The listing builds one solid part. Answer for the finished solid, in the listing's coordinates (mm). A direction names the side the tool comes from. Coordinates: 2 decimals unless noted, no trailing zeros. Order: outer loops, then holes, each group sorted by start corner. A loop starts at its lowest first (then second) coordinate and runs counter-clockwise, first axis right, second up. Notation, with made-up numbers: (85, 88.25) -> (140, 88.25) arc R25 cw to (140, 118.25) -> close; hole circle Ø8 at (64.25, 33). An arc over 180 degrees is marked (long way). Return JSON: item names as keys, results as strings.
from build123d import *

# Parameters (mm, degrees)
F1_DEPTH = 60
F2_SIZE  = 18
F4_DEPTH = 50
F6_W     = 58.8767696172
F6_H     = 9.2865563929
F7_DEPTH = 90
F8_W     = 55
F8_H     = 5
F9_DEPTH = 100


with BuildPart() as f1:
    # F0 (on Top) → F1 (new body)
    with BuildSketch(Plane.XY):
        Polygon((-16.9115909807, -35.1172805215), (16.9115909807, -35.1172805215), (38, -8.6732520268), (30.4736339606, 24.3019121461), (0, 38.9772408044), (-30.4736339606, 24.3019121461), (-38, -8.6732520268), align=None)
    extrude(amount=F1_DEPTH)

    # F2
    f2_edges = [f1.edges().sort_by_distance(p)[0] for p in [
        (0, -35.117281, 0),
        (27.455795, -21.895266, 0),
        (34.236817, 7.81433, 0),
        (15.236817, 31.639576, 0),
        (-15.236817, 31.639576, 0),
        (-34.236817, 7.81433, 0),
        (-27.455795, -21.895266, 0),
        (0, -35.117281, 60),
        (27.455795, -21.895266, 60),
        (34.236817, 7.81433, 60),
        (15.236817, 31.639576, 60),
        (-15.236817, 31.639576, 60),
        (-34.236817, 7.81433, 60),
        (-27.455795, -21.895266, 60),
    ]]
    chamfer(f2_edges, length=F2_SIZE)

    # F3 (on face) → F4 (cut)
    with BuildSketch(Plane.XY.offset(60)):
        Polygon((-18.5224097697, -4.2276191599), (-8.2432478421, -17.1172805215), (8.2432478421, -17.1172805215), (18.5224097697, -4.2276191599), (14.8538193524, 11.8455256568), (0, 18.9987480492), (-14.8538193524, 11.8455256568), align=None)
    extrude(amount=-F4_DEPTH, mode=Mode.SUBTRACT)

    # F6 (on offset) → F7 (cut)
    with BuildSketch(Plane.XZ.offset(45)):
        with Locations((0.9286543354, 60.4554843158)):
            Rectangle(F6_W, F6_H)
    extrude(amount=-F7_DEPTH, mode=Mode.SUBTRACT)

    # F8 (on offset) → F9 (cut)
    with BuildSketch(Plane.XZ.offset(45)):
        with Locations((3.5671484997, 2.5)):
            Rectangle(F8_W, F8_H)
    extrude(amount=-F9_DEPTH, mode=Mode.SUBTRACT)


solid = f1.part
1. The part is cut by section C-C on y = 7.5. Give the vertices of the cut face in (x, z).
Answer block:
{"outline": "(-34.31, 18) -> (-20.97, 5) -> (20.97, 5) -> (34.31, 18) -> (34.31, 42) -> (20.14, 55.81) -> (15.85, 55.81) -> (15.85, 10) -> (-15.85, 10) -> (-15.85, 55.81) -> (-20.14, 55.81) -> (-34.31, 42) -> close"}
2. For faces 1 (the face through (0, -17.117, 33)), 2 (the face through (22.16, -17.97, 11.41)), determine the directions among +Z, -Z, +X, -X, +Y, -Y from which every point of the face is accessible in a straight line to the end or side of a thin tool.
Answer block:
{"face 1": "+Z", "face 2": "-Z, +X, -Y"}
3. Consider line 1 (Z direction, x = -8, y = 1.5); line 2 (X direction, y = 6, z = 12); line 3 (X direction, y = 5.5, z = 16.5). Determine where each line is inside the solid, lowest interval first. Write a range as from..to.
Answer block:
{"line 1": "z = 5..10", "line 2": "x = -28.5..-16.19, 16.19..28.5", "line 3": "x = -33.23..-16.3, 16.3..33.23"}
4. The part is cut by section A-A on z = 30. Give the vertices of the cut face in (x, y), and give its area (3 significant figures).
Answer block:
{"outline": "(-38, -8.67) -> (-16.91, -35.12) -> (16.91, -35.12) -> (38, -8.67) -> (30.47, 24.3) -> (0, 38.98) -> (-30.47, 24.3) -> close; hole (-18.52, -4.23) -> (-8.24, -17.12) -> (8.24, -17.12) -> (18.52, -4.23) -> (14.85, 11.85) -> (0, 19) -> (-14.85, 11.85) -> close", "area": "3,170 mm2"}
5. Determine the mould class of faces 3 (the face through (15.45, 31.537, 29.832)), 4 (the face through (7.531, 15.372, 33.227)), 5 (the face through (0, 1, 5)) for opening direction X: pulls with the +X half, pulls with the -X half, needs draft (parallel to the pull), parting line crosses it, or undercut.
Answer block:
{"face 3": "pulls with the +X half", "face 4": "undercut", "face 5": "needs draft"}
6. The part is cut by section D-D on z = 9. Give the vertices of the cut face in (x, y).
Answer block:
{"outline": "(-28.26, -6.45) -> (-12.58, -26.12) -> (12.58, -26.12) -> (28.26, -6.45) -> (22.66, 18.07) -> (0, 28.99) -> (-22.66, 18.07) -> close"}
7. Each of these flat-tipped pins is pushed along its axis until it touches: pin 1 Ø18 at (x, y) = (-2, -4.5) entering from +Z; pin 2 Ø5 at (y, z) = (-27, 12) entering from +X; pin 3 Ø8 at (x, y) = (27.5, -22) entering from +Z. Where does it stop, or does it pass through?
Answer block:
{"pin 1": "stops at z = 10", "pin 2": "stops at x = 19.48", "pin 3": "stops at z = 45.9"}
8. The part is cut by section B-B on x = -13. Give the vertices of the cut face in (y, z).
Answer block:
{"outline": "(-35.12, 18) -> (-26.99, 9.88) -> (-19.17, 5) -> (18.29, 5) -> (32.72, 18) -> (32.72, 42) -> (17.39, 55.81) -> (12.74, 55.81) -> (12.74, 10) -> (-11.15, 10) -> (-11.15, 55.81) -> (-17.87, 55.81) -> (-26.99, 50.12) -> (-35.12, 42) -> close"}
